```python
from build123d import *

# Parameters (mm, degrees)
SKETCH1_W           = 12
SKETCH1_H           = 14
BOSS_EXTRUDE1_DEPTH = 3
SKETCH2_R           = 3.875
CUT_EXTRUDE1_DEPTH  = 3
SKETCH3_W           = 6
SKETCH3_H           = 3
BOSS_EXTRUDE2_DEPTH = 3


with BuildPart() as part:
    # Sketch1 → Boss-Extrude1 (new body)
    with BuildSketch(Plane.XY):
        with Locations((0, -1)):
            Rectangle(SKETCH1_W, SKETCH1_H)
    extrude(amount=BOSS_EXTRUDE1_DEPTH)

    # Sketch2 → Cut-Extrude1 (cut)
    with BuildSketch(Plane.XY.offset(3)):
        with Locations((0, -2)):
            Circle(SKETCH2_R)
    extrude(amount=-CUT_EXTRUDE1_DEPTH, mode=Mode.SUBTRACT)

    # Sketch3 → Boss-Extrude2 (add)
    with BuildSketch(Plane(origin=(0, 6, 0), x_dir=(1, 0, 0), z_dir=(0, 1, 0))):
        with Locations((0, -1.5)):
            Rectangle(SKETCH3_W, SKETCH3_H)
    extrude(amount=BOSS_EXTRUDE2_DEPTH)


solid = part.part
```
The model under review builds one solid part; all positions refer to its coordinate system, in mm. A direction names the side the tool comes from. Round coordinates to 2 decimals unless told otherwise and drop trailing zeros. Write each loop counter-clockwise with the first axis right and the second up, starting at its lowest first coordinate (ties: lowest second). Pieces come first, ordered by that corner, then holes.
(1) Wall thickness on L1, parallel to Y at x = 0, z = 0.85 (3 decimals); L2, parallel to Y at x = -3.5, z = 1.2; L3, parallel to X at y = -5.25, z = 1.2: over which ranges is each line inside the solid? List them lowest first.
(2) Machinability: for faces 5 (the flat face through (-6, -1, 1)), 6 (the flat face through (-5, 6, 1)), 7 (the flat face through (4, 6, 1)), which of the approach directions +Z, -Z, +X, -X, +Y, -Y give a long, thin tool a straight path to every point of the face, cutting with its end or side? Answer none if there is none.
(3) Mouldability with a two-part tool opening along Y and no side actions: class faces 1 (the cylindrical face through (-0.84, -5.783, 1.521)), 2 (the flat face through (0, -8, 1)), 3 (the flat face through (0, 3, 3)), 4 (the flat face through (0, 9, 1)) as +Y half, -Y half, draft (parallel to the pull), parting line (faces both ways), or undercut.
(4) We need section C-C on x = 1.25. Give the boundary of the cut face in (y, z), and give its area (3 significant figures).
(5) We need section B-B on z = 2.25. Give the boundary of the cut face in (x, y) (3 decimals).
(6) We need section A-A on y = -2. Give the boundary of the cut face in (x, z) (3 decimals), and give its area (4 significant figures).
(7) Insertion check: pin 1 (1.5 mm diameter, centred on x = 4.5, z = 1, fed in from +Y); pin 2 (7 mm diameter, centred on x = 0, y = -2, fed in from -Z); pin 3 (5 mm diameter, centred on x = 2.5, y = 3.5, fed in from -Z). Each pin has a flat end and moves straight along its axis. Give the tip position at first contact, or say it passes through.
(8) We need section D-D on y = 7.25. Give the boundary of the cut face in (x, z).
Findings below:
1. L1: y = -8 to -5.875, 1.875 to 9
1. L2: y = -8 to -3.66, -0.34 to 6
1. L3: x = -6 to -2.11, 2.11 to 6
2. face 5: +Z, -Z, -X, +Y, -Y
2. face 6: +Z, -Z, -X, +Y
2. face 7: +Z, -Z, +X, +Y
3. face 1: undercut
3. face 2: -Y half
3. face 3: draft
3. face 4: +Y half
4. outline: (-8, 0) - (-5.67, 0) - (-5.67, 3) - (-8, 3) - close; (1.67, 0) - (9, 0) - (9, 3) - (1.67, 3) - close
4. area: 29.0 mm2
5. outline: (-6, -8) - (6, -8) - (6, 6) - (3, 6) - (3, 9) - (-3, 9) - (-3, 6) - (-6, 6) - close; hole circle Ø7.75 at (0, -2)
6. outline: (-6, 0) - (-3.875, 0) - (-3.875, 3) - (-6, 3) - close; (3.875, 0) - (6, 0) - (6, 3) - (3.875, 3) - close
6. area: 12.75 mm2
7. pin 1: stops at y = 6
7. pin 2: passes through
7. pin 3: stops at z = 0
8. outline: (-3, 0) - (3, 0) - (3, 3) - (-3, 3) - close
